from build123d import *

# Parameters (mm, degrees)
SKETCH1_W           = 171.45
SKETCH1_H           = 50
SKETCH1_R           = 1.75
BOSS_EXTRUDE1_DEPTH = 5
CHAMFER1_SIZE       = 5
SKETCH2_W           = 139.7
SKETCH2_H           = 25.4
CUT_EXTRUDE1_DEPTH  = 2.5
SKETCH3_W           = 20.5
SKETCH3_H           = 6.5
CUT_EXTRUDE2_DEPTH  = 15


with BuildPart() as part:
    # Sketch1 → Boss-Extrude1 (new body)
    with BuildSketch(Plane(origin=(0, 0, 0), x_dir=(1, 0, 0), z_dir=(0, 1, 0))):
        Rectangle(SKETCH1_W, SKETCH1_H)
        with Locations(Location((-76.2, 17, 0), (0, 0, 270))):
            Circle(SKETCH1_R, mode=Mode.SUBTRACT)
        with Locations(Location((76.2, 17, 0), (0, 0, 270))):
            Circle(SKETCH1_R, mode=Mode.SUBTRACT)
        with Locations(Location((-76.2, -8.4, 0), (0, 0, 270))):
            Circle(SKETCH1_R, mode=Mode.SUBTRACT)
        with Locations(Location((76.2, -8.4, 0), (0, 0, 270))):
            Circle(SKETCH1_R, mode=Mode.SUBTRACT)
    extrude(amount=BOSS_EXTRUDE1_DEPTH)

    # Chamfer1
    chamfer1_edges = [part.edges().sort_by_distance(p)[0] for p in [
        (85.725, 2.5, 25),
        (-85.725, 2.5, 25),
        (-85.725, 2.5, -25),
        (85.725, 2.5, -25),
    ]]
    chamfer(chamfer1_edges, length=CHAMFER1_SIZE)

    # Sketch2 → Cut-Extrude1 (cut)
    with BuildSketch(Plane(origin=(0, 5, 0), x_dir=(1, 0, 0), z_dir=(0, 1, 0))):
        with Locations((0, 4.3)):
            Rectangle(SKETCH2_W, SKETCH2_H)
    extrude(amount=-CUT_EXTRUDE1_DEPTH, mode=Mode.SUBTRACT)

    # Sketch3 → Cut-Extrude2 (cut)
    with BuildSketch(Plane(origin=(0, 5, 0), x_dir=(1, 0, 0), z_dir=(0, 1, 0))):
        with Locations((40.55, -18.75)):
            Rectangle(SKETCH3_W, SKETCH3_H)
        with Locations((-40.55, -18.75)):
            Rectangle(SKETCH3_W, SKETCH3_H)
    extrude(amount=-CUT_EXTRUDE2_DEPTH, mode=Mode.SUBTRACT)


solid = part.part
The model under review builds one solid part; all positions refer to its coordinate system, in mm. A direction names the side the tool comes from. Round coordinates to 2 decimals unless told otherwise and drop trailing zeros. Order: outer loops, then holes, each group sorted by start corner. A loop starts at its lowest first (then second) coordinate and runs counter-clockwise, first axis right, second up. Notation, with made-up numbers: (89, 55) -> (142, 55) arc R10 ccw to (142, 62) -> close; hole circle Ø11 at (-5, 75.25). An arc over 180 degrees is marked (long way). Write item = value, one per line. Start each with the question number.
Item 1: Clearance check with flat-ended pins moving along their axes: pin 1 Ø4 at (x, z) = (-76.2, -17) entering from -Y; pin 2 Ø2 at (x, z) = (54, -13) entering from +Y; pin 3 Ø3 at (x, z) = (76.2, 8.4) entering from +Y. State where each tip first meets the part, or that it passes through.
Item 2: Consider section B-B on z = 18.5. Write out the cut boundary in (x, y) (3 decimals), plus the area to 3 significant figures.
Item 3: For line 1 along Z through (x, y) = (-31, 4.4); line 2 along Z through (x, y) = (-76.2, 2.3); line 3 along Z through (x, y) = (-48, 1.7), list the stretches that pass through material, from the lowest coordinate up.
Item 4: Consider section C-C on x = 76.2. Write out the cut boundary in (y, z).
Item 5: Mouldability with a two-part tool opening along Z and no side actions: class faces 4 (the face through (-1, 0, 0)), 5 (the face through (-41, 3, 22)), 6 (the face through (-1, 2, -25)) as released by +Z, released by -Z, zero draft, split by the parting line, or undercut.
Item 6: Consider section A-A on x = -47. Write out the cut boundary in (y, z), plus the area to 3 significant figures.
Item 7: For faces 1 (the face through (-1, 5, 11)), 2 (the face through (-1, 2.5, -4)), 3 (the face through (50.8, 3, 19)), list the 3-axis set-ups (+Z, -Z, +X, -X, +Y, -Y) from which the entire face can be reached by the end or side of a thin tool; tool diameter is ignored.
Item 8: Consider section D-D on y = 3.4. Write out the cut boundary in (x, z) (3 decimals).
Conclusion:
q1.pin_1 = 0
q1.pin_2 = 2.5
q1.pin_3 = through
q2.outline = (-85.725, 0) -> (-50.8, 0) -> (-50.8, 5) -> (-85.725, 5) -> close; (-30.3, 0) -> (30.3, 0) -> (30.3, 5) -> (-30.3, 5) -> close; (50.8, 0) -> (85.725, 0) -> (85.725, 5) -> (50.8, 5) -> close
q2.area = 652 mm2
q3.line_1 = -25 to -17, 8.4 to 15.5, 22 to 25
q3.line_2 = -25 to -18.75, -15.25 to 6.65, 10.15 to 25
q3.line_3 = -25 to 15.5, 22 to 25
q4.outline = (0, -25) -> (5, -25) -> (5, -18.75) -> (0, -18.75) -> close; (0, -15.25) -> (5, -15.25) -> (5, 6.65) -> (0, 6.65) -> close; (0, 10.15) -> (5, 10.15) -> (5, 25) -> (0, 25) -> close
q5.face_4 = zero draft
q5.face_5 = undercut
q5.face_6 = released by -Z
q6.outline = (0, -25) -> (5, -25) -> (5, -17) -> (2.5, -17) -> (2.5, 8.4) -> (5, 8.4) -> (5, 15.5) -> (0, 15.5) -> close; (0, 22) -> (5, 22) -> (5, 25) -> (0, 25) -> close
q6.area = 154 mm2
q7.face_1 = +Z, -Z, +X, -X, +Y
q7.face_2 = +Y
q7.face_3 = +Y, -Y
q8.outline = (-85.725, -20) -> (-80.725, -25) -> (80.725, -25) -> (85.725, -20) -> (85.725, 20) -> (80.725, 25) -> (-80.725, 25) -> (-85.725, 20) -> close; hole circle Ø3.5 at (-76.2, -17); hole circle Ø3.5 at (-76.2, 8.4); hole (-69.85, -17) -> (69.85, -17) -> (69.85, 8.4) -> (-69.85, 8.4) -> close; hole (-50.8, 15.5) -> (-30.3, 15.5) -> (-30.3, 22) -> (-50.8, 22) -> close; hole (30.3, 15.5) -> (50.8, 15.5) -> (50.8, 22) -> (30.3, 22) -> close; hole circle Ø3.5 at (76.2, -17); hole circle Ø3.5 at (76.2, 8.4)
